Geometry: final body of the model. Coordinates: model frame, mm. A direction names the side the tool comes from. Round coordinates to 2 decimals unless told otherwise and drop trailing zeros. Loops run counter-clockwise (first coordinate to the right, second up) from the corner with the lowest first, then second, coordinate; pieces in that order, holes last. Notation, with made-up numbers: M 45,-11 L 88,-11 A20 cw 88,1 Z; hole C 45.5,48.25 d3. An arc over 180 degrees is marked long. Answer as a JSON object with one key per item and string values.
Autodesk Inventor part; units mm, degrees
ref_plane "YZ Plane" through (0, 0, 0) normal (1, 0, 0) x (0, 1, 0)
ref_plane "XZ Plane" through (0, 0, 0) normal (0, 1, 0) x (-1, 0, 0)
ref_plane "XY Plane" through (0, 0, 0) normal (0, 0, 1) x (1, 0, 0)
sketch "Sketch1" plane through (0, 0, 0) normal (0, 1, 0) x (-1, 0, 0)
  line L0 (0, 0) -> (50, 0)
  line L1 (50, 0) -> (50, -40)
  line L2 (50, -40) -> (0, -40)
  line L3 (0, -40) -> (0, 0)
  line L4 (0, -5) -> (-20, -5)
  line L5 (-20, -5) -> (-20, -10)
  line L6 (-20, -10) -> (0, -10)
  line L7 (0, -10) -> (0, -5)
  line L8 (0, -30) -> (-20, -30)
  line L9 (-20, -30) -> (-20, -35)
  line L10 (-20, -35) -> (0, -35)
  line L11 (0, -35) -> (0, -30)
  line L12 (0, 0) -> (-3, 0)
  line L13 (-3, 0) -> (-3, -5)
  line L14 (-3, -5) -> (0, -5)
  line L15 (0, -5) -> (0, 0)
  line L16 (0, -40) -> (-3, -40)
  line L17 (-3, -40) -> (-3, -35)
  line L18 (-3, -35) -> (0, -35)
  line L19 (0, -35) -> (0, -40)
  line L20 (0, -10) -> (-3, -10)
  line L21 (-3, -10) -> (-3, -30)
  line L22 (-3, -30) -> (0, -30)
  line L23 (0, -30) -> (0, -10)
  point P0 (0, -10)
  dimension "d0" = 50
  dimension "d1" = 40
  dimension "d2" = 20
  dimension "d3" = 20
  dimension "d4" = 5
  dimension "d5" = 5
  dimension "d6" = 5
  dimension "d7" = 5
  dimension "d8" = 3
  dimension "d9" = 5
extrude "Extrusion1" add sketch "Sketch1" along normal blind 20 contours L0 L1 L2 L3 | L3 L4 L13 L12 | L3 L6 L5 L4 | L16 L17 L10 L3 | L3 L10 L9 L8
sketch "Sketch2" plane through (0, 20, 0) normal (0, 1, 0) x (1, 0, 0)
  line L0 (-50, 40) -> (-50, 0)
  line L1 (-50, 5) -> (0, 5)
  line L2 (0, 5) -> (0, 35)
  line L3 (0, 35) -> (-50, 35)
  line L4 (-50, 35) -> (-50, 5)
  line L5 (3, 40) -> (-50, 40)
  point P0 (0, 0)
  point P1 (-50, 35)
  dimension "d12" = 50
  dimension "d13" = 30
  dimension "d26" = 5
extrude "Extrusion2" cut sketch "Sketch2" against normal blind 15
sketch "Sketch3" plane through (3, 0, -5) normal (0, 0, 1) x (1, 0, 0)
  circle A0 centre (7, 10) radius 3.5
  line L0 (17, 0) -> (17, 20)
  line L1 (0, 20) -> (17, 20)
  point P0 (-3, 0)
  point P1 (8.5, 20)
  dimension "d16" = 10
  dimension "d17" = 10
  dimension "d20" = 7
extrude "Extrusion3" cut sketch "Sketch3" against normal blind 4
sketch "Sketch4" plane through (20, 0, -35) normal (0, 0, -1) x (-1, 0, 0)
  circle A0 centre (10, 10) radius 3.5
  circle A1 centre (10, 10) radius 3.5
  point P0 (20, 0)
extrude "Extrusion4" cut sketch "Sketch4" against normal blind 4
sketch "Sketch5" plane through (10, 10, -31) normal (0, 0, -1) x (-1, 0, 0)
  circle A0 centre (0, 0) radius 2
  point P0 (10, -10)
  dimension "d23" = 4
extrude "Extrusion5" cut sketch "Sketch5" against normal through all
sketch "Sketch6" plane through (0, 0, 0) normal (0, -1, 0) x (1, 0, 0)
  circle A0 centre (-37, -22.5) radius 3.5
  point P0 (0, 0)
  point P1 (-50, -5)
  point P2 (-50, -35)
  point P3 (0, -35)
  dimension "d27" = 7
  dimension "d28" = 12.5
  dimension "d29" = 37
extrude "Extrusion6" cut sketch "Sketch6" against normal blind 4
sketch "Sketch7" plane through (-37, 4, -22.5) normal (0, -1, 0) x (1, 0, 0)
  circle A0 centre (0, 0) radius 2
  point P0 (37, 22.5)
  dimension "d32" = 4
extrude "Extrusion7" cut sketch "Sketch7" against normal blind 4
properties part number "PowerSupplyAttach"
1) Reachability of faces 1 (the flat face through (-25, 13, -35)), 2 (the flat face through (14, 10, -35)), 3 (the flat face through (9.9, 7.6, -30)), 4 (the cylindrical face through (7.2, 7.9, -7)) from +Z, -Z, +X, -X, +Y, -Y: full face, straight path, thin tool, end or side. Return the list, or none.
Results:
{"face 1": "-X, +Y", "face 2": "-Z, +X, +Y, -Y", "face 3": "+X, +Y, -Y", "face 4": "+Z"}
2) Section query A-A (z = -22.5). Return the cut outline in (x, y).
Results:
{"outline": "M -50,0 L -40.5,0 L -40.5,4 L -39,4 L -39,5 L -50,5 Z; M -35,4 L -33.5,4 L -33.5,0 L 0,0 L 0,5 L -35,5 Z"}
3) Section query D-D (x = -37). Return the cut outline in (y, z).
Results:
{"outline": "M 0,-40 L 20,-40 L 20,-35 L 5,-35 L 5,-24.5 L 4,-24.5 L 4,-26 L 0,-26 Z; M 0,-19 L 4,-19 L 4,-20.5 L 5,-20.5 L 5,-5 L 20,-5 L 20,0 L 0,0 Z"}
4) Section query B-B (y = 19). Return the cut outline in (x, z), and give its area (3 significant figures).
Results:
{"outline": "M -50,-40 L 3,-40 L 3,-35 L 20,-35 L 20,-30 L 0,-30 L 0,-35 L -50,-35 Z; M -50,-5 L 0,-5 L 0,-10 L 20,-10 L 20,-5 L 3,-5 L 3,0 L -50,0 Z", "area": "730 mm2"}
5) Section query C-C (x = 10). Return the cut outline in (y, z).
Results:
{"outline": "M 0,-35 L 6.5,-35 L 6.5,-31 L 8,-31 L 8,-30 L 0,-30 Z; M 0,-10 L 8,-10 L 8,-9 L 6.5,-9 L 6.5,-5 L 0,-5 Z; M 12,-31 L 13.5,-31 L 13.5,-35 L 20,-35 L 20,-30 L 12,-30 Z; M 12,-10 L 20,-10 L 20,-5 L 13.5,-5 L 13.5,-9 L 12,-9 Z"}
6) Pin query (flat end, axial travel): P1, Ø12, axis at x = 9, z = -35.5, coming from the +Y side; P2, Ø5.5, axis at y = 14.5, z = -2, coming from the +X side; P3, Ø6.5, axis at x = -37, z = -22.5, coming from the +Y side; P4, Ø5.5, axis at x = 8.5, y = 11, coming from the +Z side. Return the tip coordinate at first contact, or that it passes through.
Results:
{"P1": "y = 20", "P2": "x = 3", "P3": "y = 5", "P4": "z = -5"}
7) Pull-direction query (X, two-part tool) for faces 5 (the flat face through (0, 13, -32)), 6 (the flat face through (13.3, 7.6, -5)), 7 (the cylindrical face through (10.26, 11.983, -30.507)), 8 (the cylindrical face through (10.26, 11.983, -9.507)); classes: +X half, -X half, draft (parallel to the pull), parting line (faces both ways), or undercut.
Results:
{"face 5": "-X half", "face 6": "draft", "face 7": "undercut", "face 8": "undercut"}
8) Ray query, line 1 (Y direction, x = 10, z = -9.45); line 2 (Z direction, x = -39.5, y = 5.25); line 3 (Z direction, x = 7.5, y = 16). Return the intervals inside material, ascending.
Results:
{"line 1": "0 to 8, 12 to 20", "line 2": "-40 to -35, -5 to 0", "line 3": "-35 to -30, -10 to -5"}
